The model under review builds one solid part; all positions refer to its coordinate system, in mm. Face numbers are marked on the shaded views. Coordinates: 2 decimals unless noted, no trailing zeros. Write each loop counter-clockwise with the first axis right and the second up, starting at its lowest first coordinate (ties: lowest second). Pieces come first, ordered by that corner, then holes.
1) Add section A-A, the plane x = 5. Give the number of separate pieces and of enclosed holes in the cut face, then the cut area to 3 significant figures.
2) Mouldability with a two-part tool opening along Z and no side actions: class the marked faces 1, 2 and 3 as released by +Z, released by -Z, zero draft, split by the parting line, or undercut.
3) For P1, Ø5.5, axis at x = 5, z = 3, coming from the +Y side, flat-tipped, find the tip position at first contact; note if it passes through.
4) For line 1 (Z direction, x = -5, y = 4); line 2 (Z direction, x = 2.25, y = 6.5); line 3 (Z direction, x = 8.25, y = 4.75), list the stretches that pass through material, from the lowest coordinate up.
5) Add section B-B, the plane y = 4.5. State the section outline as (x, z) points.
6) Add section D-D, the plane z = 3. State the section outline as (x, y) points, then the cut area to 3 significant figures.
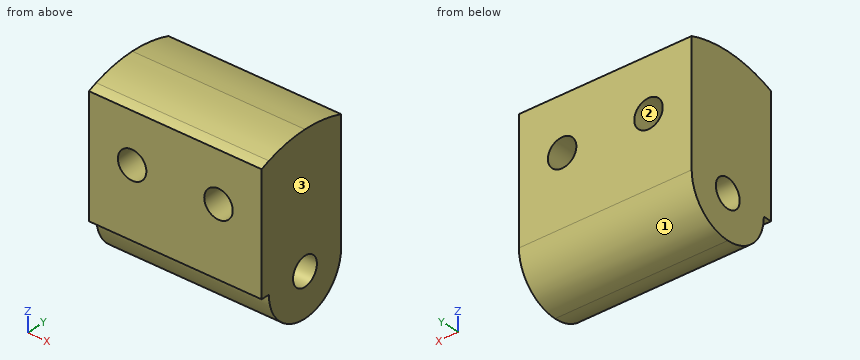
from build123d import *

# Parameters (mm, degrees)
SKETCH1_W             = 20
SKETCH1_H             = 20
BOSS_EXTRUDE1_DEPTH   = 10
FILLET1_R             = 5
M4X0_7_TAPPED_HOLE1_D = 3.3
SKETCH14_W            = 20
SKETCH14_H            = 15
BOSS_EXTRUDE4_DEPTH   = 1
M4X0_7_TAPPED_HOLE2_D = 3.3
CUT_EXTRUDE1_DEPTH    = 25.494897428


with BuildPart() as part:
    # Sketch1 → Boss-Extrude1 (new body)
    with BuildSketch(Plane(origin=(0, 0, 0), x_dir=(1, 0, 0), z_dir=(0, 1, 0))):
        Rectangle(SKETCH1_W, SKETCH1_H)
    extrude(amount=BOSS_EXTRUDE1_DEPTH)

    # Fillet1
    fillet1_edges = [part.edges().sort_by_distance(p)[0] for p in [
        (0, 0, -10),
        (0, 10, -10),
    ]]
    fillet(fillet1_edges, radius=FILLET1_R - 0.0001)  # a hair under: the kernel refuses the full size

    # M4x0.7 Tapped Hole1 (through all)
    with Locations(Plane(origin=(10, 0, 0), x_dir=(0, 0, -1), z_dir=(1, 0, 0))):
        with Locations((5, 5)):
            Hole(M4X0_7_TAPPED_HOLE1_D / 2)

    # Sketch14 → Boss-Extrude4 (add)
    with BuildSketch(Plane.XZ):
        with Locations((0, 2.5)):
            Rectangle(SKETCH14_W, SKETCH14_H)
    extrude(amount=BOSS_EXTRUDE4_DEPTH)

    # M4x0.7 Tapped Hole2 (through all)
    with Locations(Plane(origin=(0, 10, 0), x_dir=(1, 0, 0), z_dir=(0, 1, 0))):
        with Locations((-5, -3), (5, -3)):
            Hole(M4X0_7_TAPPED_HOLE2_D / 2)

    # Sketch9 → Cut-Extrude1 (cut, through all)
    with BuildSketch(Plane(origin=(10, 0, 0), x_dir=(0, 0, -1), z_dir=(1, 0, 0))):
        with BuildLine():
            ThreePointArc((-10, 5), (-9.783978395, 7.536529681), (-9.142135624, 10))
            Line((-9.142135624, 10), (-10, 10))
            Line((-10, 10), (-10, 5))
        make_face()
        with BuildLine():
            Line((-10, 0), (-9.142135624, 0))
            ThreePointArc((-9.142135624, 0), (-9.783978395, 2.463470319), (-10, 5))
            Line((-10, 5), (-10, 0))
        make_face()
        with BuildLine():
            Line((-10, -1), (-8.747727085, -1))
            ThreePointArc((-8.747727085, -1), (-8.953892306, -0.503534276), (-9.142135624, 0))
            Line((-9.142135624, 0), (-10, 0))
            Line((-10, 0), (-10, -1))
        make_face()
    extrude(amount=-CUT_EXTRUDE1_DEPTH, mode=Mode.SUBTRACT)


solid = part.part
Geometry results:
1. separate pieces: 2
1. enclosed holes: 1
1. area: 156 mm2
2. face 1: released by -Z
2. face 2: undercut
2. face 3: zero draft
3. P1: stops at y = 10
4. line 1: z = -9.9 to -6.31, -3.69 to 1.35, 4.65 to 9.97
4. line 2: z = -9.77 to -5.69, -4.31 to 9.92
4. line 3: z = -9.99 to -6.63, -3.37 to 10
5. outline: (-10, -9.97) - (10, -9.97) - (10, -6.57) - (-10, -6.57) - close; (-10, -3.43) - (10, -3.43) - (10, 9.99) - (-10, 9.99) - close; hole circle Ø3.3 at (-5, 3); hole circle Ø3.3 at (5, 3)
6. outline: (-10, -1) - (-6.65, -1) - (-6.65, 10) - (-10, 10) - close; (-3.35, -1) - (3.35, -1) - (3.35, 10) - (-3.35, 10) - close; (6.65, -1) - (10, -1) - (10, 10) - (6.65, 10) - close
6. area: 147 mm2
